Geometry: final body of the model. Coordinates: model frame, mm. Face numbers are marked on the shaded views. Round coordinates to 2 decimals unless told otherwise and drop trailing zeros. Loops run counter-clockwise (first coordinate to the right, second up) from the corner with the lowest first, then second, coordinate; pieces in that order, holes last. Notation, with made-up numbers: (38.25, 36.5) - (62.25, 36.5) arc R13 ccw to (62.25, 53.5) - close; hole circle Ø10 at (-3.5, -3.5). An arc over 180 degrees is marked (long way). Answer as CSV lines item,"result".
from build123d import *


with BuildPart() as part:
    # Sketch1 → Revolve1 (revolve)
    with BuildSketch(Plane.XY, mode=Mode.PRIVATE) as revolve1_sk:
        with BuildLine():
            ThreePointArc((0, 1.25), (-0.057874055, 1.58525916), (-0.224797408, 1.881712705))
            Line((-0.224797408, 1.881712705), (-0.03099676, 2.039640881))
            ThreePointArc((-0.03099676, 2.039640881), (0.177657431, 1.66907395), (0.25, 1.25))
            Line((0.25, 1.25), (0.25, 1))
            Line((0.25, 1), (0, 1))
            Line((0, 1), (-2, 1))
            Line((-2, 1), (-2.25, 1))
            ThreePointArc((-2.25, 1), (-2.284841337, 1.897834477), (-2, 2.75))
            Line((-2, 2.75), (-1.78099676, 2.629428109))
            ThreePointArc((-1.78099676, 2.629428109), (-2.021139042, 1.960479194), (-2.040639843, 1.25))
            Line((-2.040639843, 1.25), (0, 1.25))
        make_face()
    revolve(revolve1_sk.sketch.rotate(Axis((0, 0, 0), (-1, 0, 0)), 90), axis=Axis((0, 0, 0), (-1, 0, 0)))


solid = part.part
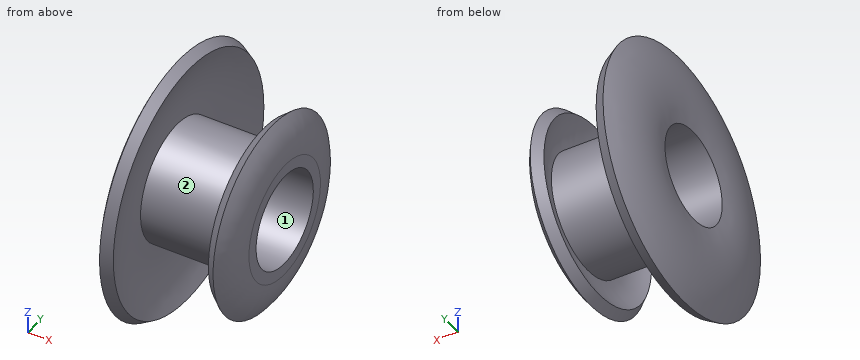
(1) Section A-A (x = -0.6). Output: boundary loops of the cut face in (y, z), and give its area (3 significant figures).
Findings below:
outline,"circle Ø2.5 at (0, 0); hole circle Ø2 at (0, 0)"
area,"1.77 mm2"
(2) Draft query along X for the marked faces 1 and 2. Return one class per face: pulls with the +X half, pulls with the -X half, needs draft (parallel to the pull), parting line crosses it, or undercut.
Findings below:
face 1,"needs draft"
face 2,"undercut"
(3) Material intervals for line 1 along Y through (x, z) = (-0.35, 0); line 2 along Z through (x, y) = (-1, 0.65); line 3 along Z through (x, y) = (-1.75, 0.7), sorted ascending.
Findings below:
line 1,"-1.25 to -1, 1 to 1.25"
line 2,"-1.07 to -0.76, 0.76 to 1.07"
line 3,"-1.04 to -0.71, 0.71 to 1.04"
(4) Pin query (flat end, axial travel): P1, Ø2, axis at y = -1.5, z = 1.5, coming from the -X side; P2, Ø1.6, axis at y = 0, z = 0, coming from the +X side. Return the tip coordinate at first contact, or that it passes through.
Findings below:
P1,"x = -2.31"
P2,"through"
(5) Section B-B (x = -0.1). Output: boundary loops of the cut face in (y, z), and give its area (3 significant figures).
Findings below:
outline,"circle Ø3.97 at (0, 0); circle Ø2.5 at (0, 0); hole circle Ø3.37 at (0, 0); hole circle Ø2 at (0, 0)"
area,"5.20 mm2"
